from build123d import *

# Parameters (mm, degrees)
SKETCH_1_W          = 73
SKETCH_1_H          = 3
EXTRUDE_1_DEPTH     = 20
SKETCH_2_R          = 1.25
SKETCH_2_R_2        = 2
CUT_EXTRUDE_1_DEPTH = 20
FILLET_1_R          = 2


with BuildPart() as part:
    # Эскиз1 → Бобышка-Вытянуть1 (new body)
    with BuildSketch(Plane(origin=(0, 0, 0), x_dir=(1, 0, 0), z_dir=(0, 1, 0))):
        with Locations((204.810975887, -13.655372437)):
            Rectangle(SKETCH_1_W, SKETCH_1_H)
    extrude(amount=EXTRUDE_1_DEPTH)

    # Эскиз2 → Вырез-Вытянуть1 (cut)
    with BuildSketch(Plane(origin=(0, 0, 12.155372437), x_dir=(-1, 0, 0), z_dir=(0, 0, -1))):
        with Locations((-173.310975887, 15)):
            Circle(SKETCH_2_R)
        with Locations((-183.310975887, 10)):
            Circle(SKETCH_2_R)
        with Locations((-173.310975887, 5)):
            Circle(SKETCH_2_R)
        with Locations((-236.510975887, 10)):
            Circle(SKETCH_2_R_2)
        with Locations((-194.510975887, 15)):
            Circle(SKETCH_2_R)
        with Locations(Location((-194.510975887, 5, 0), (0, 0, 180))):
            Circle(SKETCH_2_R)
        with Locations((-226.510975887, 15)):
            Circle(SKETCH_2_R)
        with Locations(Location((-226.510975887, 5, 0), (0, 0, 180))):
            Circle(SKETCH_2_R)
    extrude(amount=-CUT_EXTRUDE_1_DEPTH, mode=Mode.SUBTRACT)

    # Скругление1
    fillet_1_edges = [part.edges().sort_by_distance(p)[0] for p in [
        (241.310975887, 10, 12.155372437),
    ]]
    fillet(fillet_1_edges, radius=FILLET_1_R)


solid = part.part
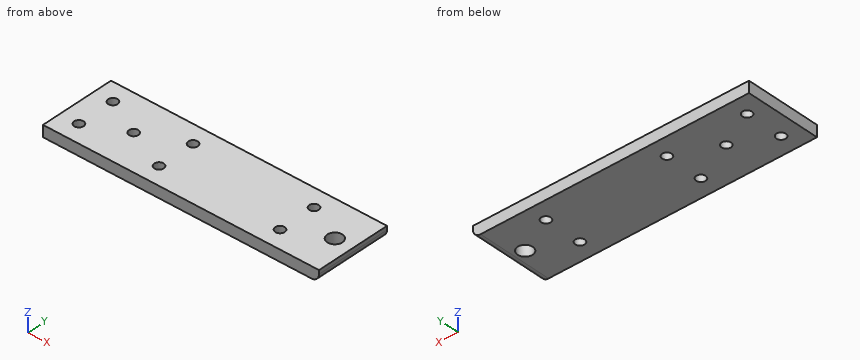
Read the model definition and answer for the solid it produces. Units are mm, in the model's axes. Round coordinates to 2 decimals unless told otherwise and drop trailing zeros. Loops run counter-clockwise (first coordinate to the right, second up) from the corner with the lowest first, then second, coordinate; pieces in that order, holes last.
Q1. Section B-B on z = 13.65 is taken. Give the number of separate pieces and of enclosed holes in the cut face, and give its area (3 significant figures).
Q2. Section A-A on y = 5 is taken. Write down the section's boundary in (x, z).
Q3. Section C-C on y = 10 is taken. Write down the section's boundary in (x, z), and give its area (3 significant figures).
Q4. Consider probe 1 along Y at (x, z) = (226.5, 13.95); probe 2 along Y at (x, z) = (172.5, 14.7); probe 3 along X at (y, z) = (9.25, 12.8). Determine where each line is inside the solid, lowest interval first.
Output:
1. separate pieces: 1
1. enclosed holes: 8
1. area: 1,410 mm2
2. outline: (168.31, 12.16) - (172.06, 12.16) - (172.06, 15.16) - (168.31, 15.16) - close; (174.56, 12.16) - (193.26, 12.16) - (193.26, 15.16) - (174.56, 15.16) - close; (195.76, 12.16) - (225.26, 12.16) - (225.26, 15.16) - (195.76, 15.16) - close; (227.76, 12.16) - (239.31, 12.16) arc R2 ccw to (241.31, 14.16) - (241.31, 15.16) - (227.76, 15.16) - close
3. outline: (168.31, 12.16) - (182.06, 12.16) - (182.06, 15.16) - (168.31, 15.16) - close; (184.56, 12.16) - (234.51, 12.16) - (234.51, 15.16) - (184.56, 15.16) - close; (238.51, 12.16) - (239.31, 12.16) arc R2 ccw to (241.31, 14.16) - (241.31, 15.16) - (238.51, 15.16) - close
3. area: 199 mm2
4. probe 1: y = 0 to 3.75, 6.25 to 13.75, 16.25 to 20
4. probe 2: y = 0 to 4.05, 5.95 to 14.05, 15.95 to 20
4. probe 3: x = 168.31 to 182.31, 184.31 to 234.66, 238.37 to 240.78
